Verification items for the finished model (mm, model axes). Coordinates: 2 decimals unless noted, no trailing zeros. Write each loop counter-clockwise with the first axis right and the second up, starting at its lowest first coordinate (ties: lowest second). Pieces come first, ordered by that corner, then holes.
Autodesk Inventor part; units mm, degrees
ref_plane "Start Plane" through (0, 0, -15) normal (0, 0, 1) x (1, 0, 0)
ref_plane "End Plane" through (0, 0, 785) normal (0, 0, 1) x (1, 0, 0)
ref_plane "Work Plane4" through (0, 15, -15) normal (0, -0.7071, -0.7071) x (1, 0, 0)
ref_plane "Start Plane" through (0, 0, -15) normal (0, 0, 1) x (1, 0, 0)
ref_plane "End Plane" through (0, 0, 785) normal (0, 0, 1) x (1, 0, 0)
sketch "Sketch" plane through (0, 0, 0) normal (0, 0, 1) x (1, 0, 0)
  line L0 (-15, -9) -> (-15, 9)
  line L1 (-9, 15) -> (9, 15)
  line L2 (15, 9) -> (15, -9)
  line L3 (9, -15) -> (-9, -15)
  arc A0 (-15, -9) -> (-9, -15) centre (-9, -9) ccw
  arc A1 (-9, 15) -> (-15, 9) centre (-9, 9) ccw
  arc A2 (15, 9) -> (9, 15) centre (9, 9) ccw
  arc A3 (9, -15) -> (15, -9) centre (9, -9) ccw
  arc A4 (-9, 12) -> (-12, 9) centre (-9, 9) ccw
  line L4 (-9, 12) -> (9, 12)
  arc A5 (12, 9) -> (9, 12) centre (9, 9) ccw
  line L5 (12, 9) -> (12, -9)
  arc A6 (9, -12) -> (12, -9) centre (9, -9) ccw
  line L6 (9, -12) -> (-9, -12)
  arc A7 (-12, -9) -> (-9, -12) centre (-9, -9) ccw
  line L7 (-12, -9) -> (-12, 9)
  line L8 (0, 22.7397) -> (0, -22.7397) construction
  line L9 (-22.7397, 0) -> (22.7397, 0) construction
  dimension "d7" = 6
  dimension "d10" = 30
  dimension "d11" = 30
  dimension "d12" = 3
  dimension "d15" = 15
  dimension "d16" = 15
extrude "Body" add sketch "Sketch" along normal up to surface (800 mm away) from surface at -15
sketch "Sketch3" plane through (0, 0, 0) normal (0, 0, 1) x (1, 0, 0)
  line L0 (0, 0) -> (10, 0)
ref_plane "Work Plane3" through (0, 0, 0) normal (0, -1, 0) x (1, 0, 0)
ref_plane "Work Plane4" through (0, 15, -15) normal (0, -0.7071, -0.7071) x (1, 0, 0)
split "Split1" plane through (0, 15, -15) removes the side toward (0, -0.7071, -0.7071)
ref_plane "Work Plane5" through (9, 500, 785) normal (0, 0, 1) x (1, 0, 0)
split "Split2" plane through (9, 500, 785) removes the side toward (0, 0, 1)
sketch "Sketch4" plane through (0, 0, 0) normal (0, -1, 0) x (1, 0, 0)
  line L0 (-2, -15) -> (12, -15)
  line L1 (-2, 785) -> (12, 785)
  dimension "d18" = 800
equation "\"d7\" = G_IR"
equation "\"d10\" = G_H"
equation "\"d11\" = G_W"
equation "\"d12\" = G_T"
equation "\"d15\" = 0.5 * d10"
equation "\"d16\" = 0.5 * d11"
equation "\"d3\" = G_L"
equation "\"G_W\" = 30"
equation "\"G_H\" = 30"
equation "\"G_T\" = 3"
equation "\"G_IR\" = 6"
equation "\"G_L\" = d18"
equation "\"G_OFFSET_START\" = 15"
equation "\"G_OFFSET_END\" = -15"
equation "\"d13\" = -G_OFFSET_START"
equation "\"d14\" = G_OFFSET_END + B_L"
properties part number "DIN EN 10219-2 - 30 x 30 x 3  - 800" material "Steel, Mild"
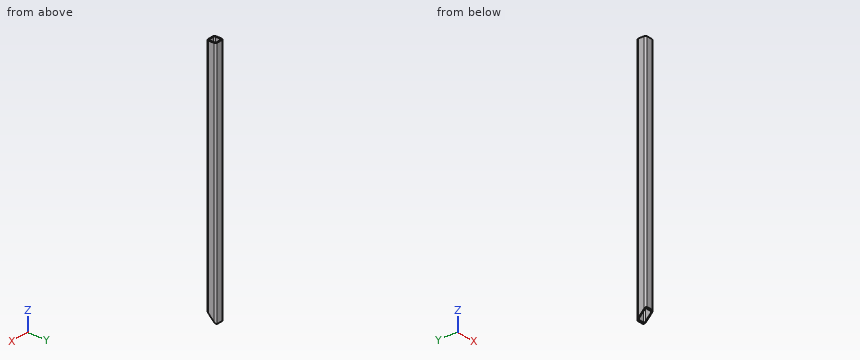
1. Material ranges on L1, parallel to Y at x = -4.5, z = 127; L2, parallel to Y at x = -11.75, z = 154.5, recorded low to high.
2. Sectioned sample at C-C, the plane y = -2.5. Record the boundary of the cut face in (x, z), and give its area (4 significant figures).
3. Sectioned sample at B-B, the plane z = 289.5. Record the boundary of the cut face in (x, y).
4. Gauge pin test, flat ends, axial feed: P1, Ø6, axis at x = 9.5, z = 661, coming from the +Y side; P2, Ø4, axis at x = 7.5, y = 12, coming from the -Z side. Record the tip position at first contact, or that the pin passes through.
5. Sectioned sample at A-A, the plane x = -2.25. Record the boundary of the cut face in (y, z), and give its area (3 significant figures).
Outcome:
1. L1: y = -15 to -12, 12 to 15
1. L2: y = -14.33 to -10.2, 10.2 to 14.33
2. outline: (-15, 2.5) - (-12, 2.5) - (-12, 785) - (-15, 785) - close; (12, 2.5) - (15, 2.5) - (15, 785) - (12, 785) - close
2. area: 4,695 mm2
3. outline: (-15, -9) arc R6 ccw to (-9, -15) - (9, -15) arc R6 ccw to (15, -9) - (15, 9) arc R6 ccw to (9, 15) - (-9, 15) arc R6 ccw to (-15, 9) - close; hole (-12, -9) arc R3 ccw to (-9, -12) - (9, -12) arc R3 ccw to (12, -9) - (12, 9) arc R3 ccw to (9, 12) - (-9, 12) arc R3 ccw to (-12, 9) - close
4. P1: stops at y = 15
4. P2: stops at z = -14
5. outline: (-15, 15) - (-12, 12) - (-12, 785) - (-15, 785) - close; (12, -12) - (15, -15) - (15, 785) - (12, 785) - close
5. area: 4,710 mm2
